```python
from build123d import *

# Parameters (mm, degrees)
ESTRUSIONE_ESTRUSIONE2_DEPTH = 6
SMUSSO1_SIZE                 = 1
RACCORDO5_R                  = 1.707107


# Read off the part's stored shape, not the designer's step: Estrusione-Estrusione2
with BuildPart() as part:
    # Estrusione-Estrusione2 outline → Estrusione-Estrusione2 (new body)
    with BuildSketch(Plane.XY):
        with BuildLine():
            Line((-54.136250947, 19.470330923), (-54.136250947, 17.522149798))
            Line((-54.136250947, 17.522149798), (-51.559423685, 17.522149798))
            ThreePointArc((-51.559423685, 17.522149798), (-50.228448587, 15.523864916), (-49.484742197, 13.240985597))
            Line((-49.484742197, 13.240985597), (-59.687524076, -14.833797153))
            ThreePointArc((-59.687524076, -14.833797153), (-59.02122155, -18.875711178), (-55.222335236, -20.408516065))
            Line((-55.222335236, -20.408516065), (-55.222335236, -19.277551448))
            ThreePointArc((-55.222335236, -19.277551448), (-57.864636062, -17.890294899), (-58.223117797, -14.927572295))
            Line((-58.223117797, -14.927572295), (-47.522213123, 13.240985597))
            ThreePointArc((-47.522213123, 13.240985597), (-48.637151321, 16.732148519), (-51.073062414, 19.470330923))
            Line((-51.073062414, 19.470330923), (-54.136250947, 19.470330923))
        make_face()
    extrude(amount=ESTRUSIONE_ESTRUSIONE2_DEPTH)

    # Smusso1
    smusso1_edges = [part.edges().sort_by_distance(p)[0] for p in [
        (-54.136250947, 19.470330923, 3),
    ]]
    chamfer(smusso1_edges, length=SMUSSO1_SIZE)

    # Raccordo5
    raccordo5_edges = [part.edges().sort_by_distance(p)[0] for p in [
        (-54.136250947, 18.470330923, 3),
        (-53.136250947, 19.470330923, 3),
    ]]
    fillet(raccordo5_edges, radius=RACCORDO5_R - 0.0001)  # a hair under: the kernel refuses the full size


solid = part.part
```
CAD build for the part. Positions are in the model's coordinates, mm. A direction names the side the tool comes from. Give positions to 0.01 mm unless a question says otherwise; leave off trailing zeros. Order: outer loops, then holes, each group sorted by start corner. A loop starts at its lowest first (then second) coordinate and runs counter-clockwise, first axis right, second up.
(1) Tool access for faces 4 (the cylindrical face through (-50.24, 15.55, 2.96)), 5 (the flat face through (-52, 19.47, 3)), 6 (the flat face through (-55.222, -20, 3)), 7 (the flat face through (-52.948, -1.04, 2.958)): list every direction of +Z, -Z, +X, -X, +Y, -Y with a clear straight run to the whole face (end or side of a thin tool).
(2) Saw through at D-D, the plane x = -49. Give the cut face in (y, z), then the cut area to 3 significant figures.
(3) Drill centre lines: L1, parallel to X at y = 0.5, z = 1.4 (3 decimals); L2, parallel to X at y = -10, z = 2.3. Where is each one in solid material? Low to high.
(4) Saw through at C-C, the plane y = -2. Give the cut face in (x, z), then the cut area to 3 significant figures.
(5) Saw through at A-A, the plane x = -50.5. Give the cut face in (y, z).
(6) Mould opens along Y. For faces 1 (the cylindrical face through (-54.01, 18.41, 3.04)), 2 (the flat face through (-54.515, -0.6, 2.958)), 3 (the flat face through (-53, 1, 0)) say: released by +Y, released by -Y, zero draft, split by the parting line, or undercut.
(7) Flat gauge pins, fed straight in: pin 1 (1.2 mm diameter, centred on y = -20, z = 2, fed in from +X); pin 2 (1 mm diameter, centred on y = -9, z = 5, fed in from -X); pin 3 (2 mm diameter, centred on y = 12, z = 4.5, fed in from -X). Where does each tip first touch, or does it go through?
Results found:
1. face 4: +Z, -Z, -X
1. face 5: +Z, -Z, +X, -X, +Y
1. face 6: +Z, -Z, +X, -Y
1. face 7: +Z, -Z, +X
2. outline: (9.35, 0) - (17.31, 0) - (17.31, 6) - (9.35, 6) - close
2. area: 47.8 mm2
3. L1: x = -54.115 to -52.362
3. L2: x = -57.93 to -56.35
4. outline: (-55.02, 0) - (-53.31, 0) - (-53.31, 6) - (-55.02, 6) - close
4. area: 10.3 mm2
5. outline: (5.4, 0) - (10.45, 0) - (10.45, 6) - (5.4, 6) - close; (16.04, 0) - (19.01, 0) - (19.01, 6) - (16.04, 6) - close
6. face 1: released by +Y
6. face 2: undercut
6. face 3: zero draft
7. pin 1: stops at x = -55.22
7. pin 2: stops at x = -57.75
7. pin 3: stops at x = -50.3
